```python
from build123d import *

# Parameters (mm, degrees)
F1_DEPTH = 27
F4_DEPTH = 29.13629
F5_W     = 556.250348
F5_H     = 232.422799
F6_DEPTH = 50


with BuildPart() as f1:
    # F0 (on Top) → F1 (new body)
    with BuildSketch(Plane.XY):
        with BuildLine():
            ThreePointArc((103.141751, 130.827628), (147.000525, 190.646497), (220.000119, 203.797485))
            Line((220.000119, 203.797485), (331.982739, 180.898076))
            ThreePointArc((331.982739, 180.898076), (297.759937, 202.019334), (260.019282, 215.909999))
            ThreePointArc((260.019282, 215.909999), (247.785722, 214.790312), (240.327458, 224.551869))
            ThreePointArc((240.327458, 224.551869), (186.047212, 230.450127), (134.405585, 212.722269))
            ThreePointArc((134.405585, 212.722269), (96.675345, 191.925026), (57.181264, 174.711255))
            ThreePointArc((57.181264, 174.711255), (38.789615, 163.844419), (25.042325, 147.493489))
            ThreePointArc((25.042325, 147.493489), (-75.160431, 14.302014), (-203.064791, -92.567234))
            ThreePointArc((-203.064791, -92.567234), (-248.600788, -164.483519), (-272.445342, -246.19592))
            Line((-272.445342, -246.19592), (-253.424359, -365.238374))
            ThreePointArc((-253.424359, -365.238374), (-248.03197, -364.036727), (-243.660012, -360.659182))
            ThreePointArc((-243.660012, -360.659182), (-226.474264, -324.191868), (-229.146522, -283.966577))
            ThreePointArc((-229.146522, -283.966577), (-222.505303, -205.585554), (-161.231884, -156.257483))
            ThreePointArc((-161.231884, -156.257483), (-11.343038, -29.016538), (103.141751, 130.827628))
        make_face()
    extrude(amount=F1_DEPTH)

    # F3 (on face) → F4 (cut)
    with BuildSketch(Plane.XY.offset(27)):
        with BuildLine():
            ThreePointArc((-240.724359, -352.538374), (-262.404616, -343.558118), (-253.424359, -365.238374))
            ThreePointArc((-253.424359, -365.238374), (-248.03197, -364.036727), (-243.660012, -360.659182))
            ThreePointArc((-243.660012, -360.659182), (-241.4808, -356.855942), (-240.724359, -352.538374))
        make_face()
    extrude(amount=-F4_DEPTH, mode=Mode.SUBTRACT)

    # F5 (on face) → F6 (cut)
    with BuildSketch(Plane.XY):
        with Locations((93.210183, 116.211399)):
            Rectangle(F5_W, F5_H)
    extrude(amount=F6_DEPTH, mode=Mode.SUBTRACT)


solid = f1.part
```
CAD build for the part. Positions are in the model's coordinates, mm. Coordinates: 2 decimals unless noted, no trailing zeros. Loops run counter-clockwise (first coordinate to the right, second up) from the corner with the lowest first, then second, coordinate; pieces in that order, holes last. Notation, with made-up numbers: (24, -22) - (28, -22) arc R25 cw to (28, 17) - close; hole circle Ø5 at (2.25, -8). An arc over 180 degrees is marked (long way). Return JSON: item names as keys, results as strings.
1. Mould opens along Y. For faces 1 (the cylindrical face through (-248.107, -163.395, 13.311)), 2 (the cylindrical face through (-226.58, -324.75, 13.31)), 3 (the cylindrical face through (-69.05, -85.67, 13.31)), 4 (the cylindrical face through (-223.03, -206.59, 13.31)) say: released by +Y, released by -Y, zero draft, split by the parting line, or undercut.
Result:
{"face 1": "released by +Y", "face 2": "undercut", "face 3": "released by -Y", "face 4": "undercut"}
2. Band-saw the part on B-B (x = -247.5). Give the cut face in (y, z).
Result:
{"outline": "(-341.3, 0) - (-162.07, 0) - (-162.07, 27) - (-341.3, 27) - close"}
3. Band-saw the part on A-A (z = 17). Give the cut face in (x, y).
Result:
{"outline": "(-272.45, -246.2) - (-257.38, -340.47) arc R12.7 cw to (-240.72, -352.54) arc R12.7 cw to (-243.66, -360.66) arc R80.41 ccw to (-229.15, -283.97) arc R100 cw to (-161.23, -156.26) arc R803.19 ccw to (14.12, 0) - (-89.13, 0) arc R726.99 cw to (-203.06, -92.57) arc R304.42 ccw to start"}
4. Band-saw the part on C-C (y = -147.5). Give the cut face in (x, z), and give its area (3 significant figures).
Result:
{"outline": "(-240.29, 0) - (-148.18, 0) - (-148.18, 27) - (-240.29, 27) - close", "area": "2,490 mm2"}
5. Drop flat-ended pins along their axis: pin 1 (1 mm diameter, centred on x = -196, z = 7, fed in from +Y); pin 2 (4 mm diameter, centred on x = -175, y = -95, fed in from -Z); pin 3 (8 mm diameter, centred on x = -173.5, z = 6.5, fed in from +Y); pin 4 (1.5 mm diameter, centred on x = -120, z = 16.5, fed in from -Y). Give the stop position or say it passes through.
Result:
{"pin 1": "stops at y = -87.53", "pin 2": "stops at z = 0", "pin 3": "stops at y = -69.14", "pin 4": "stops at y = -127.85"}
6. Probe L1, parallel to Y at x = -242, z = 15.5; L2, parallel to X at y = -299, z = 18.5; L3, parallel to X at y = -239, z = 22.5. List the from-to ranges inside material, lowest first. Write a range as from..to.
Result:
{"L1": "y = -358.59..-358.09, -346.99..-150.79", "L2": "x = -264.01..-225.73", "L3": "x = -271.32..-233.29"}
